The listing builds one solid part. Answer for the finished solid, in the listing's coordinates (mm). Face numbers are marked on the shaded views. A direction names the side the tool comes from. Round coordinates to 2 decimals unless told otherwise and drop trailing zeros. Order: outer loops, then holes, each group sorted by start corner. A loop starts at its lowest first (then second) coordinate and runs counter-clockwise, first axis right, second up. Notation, with made-up numbers: (-21, 37) -> (-15, 37) arc R15 cw to (-15, 50) -> close; hole circle Ø9 at (11, -11). An arc over 180 degrees is marked (long way). Return JSON: item names as keys, results as strings. Group by question number.
(1) The part is cut by section B-B (y = -31). Determine the outline of the cut face in (x, z), plus the area to 3 significant figures.
(2) The part is cut by section D-D (z = 30.5). Determine the outline of the cut face in (x, y).
(3) Consider line 1 (Y direction, x = -22, z = 69.5); line 2 (X direction, y = -21, z = 44.5); line 3 (X direction, y = -56, z = 28.5). Determine where each line is inside the solid, lowest interval first. Write a range as [from, to].
(4) Which of the six approach directions +Z, -Z, +X, -X, +Y, -Y give full straight-line access (tool end or side, diameter ignored) to the marked faces 1 and 2?
(5) The part is cut by section C-C (x = -68). Determine the outline of the cut face in (y, z).
(6) The part is cut by section A-A (z = 38.5). Determine the outline of the cut face in (x, y).
(7) Each of these flat-tipped pins is pushed along its axis until it touches: pin 1 (16 mm diameter, centred on y = -53.5, z = 12.5, fed in from +X); pin 2 (10 mm diameter, centred on x = -61, y = -29.5, fed in from +Z); pin 3 (1 mm diameter, centred on y = -39, z = 10, fed in from +X). Where does it stop, or does it pass through?
(8) Determine the mould class of the marked faces 3, 4, 5 and 6 for opening direction Z: +Z half, -Z half, draft (parallel to the pull), parting line (faces both ways), or undercut.
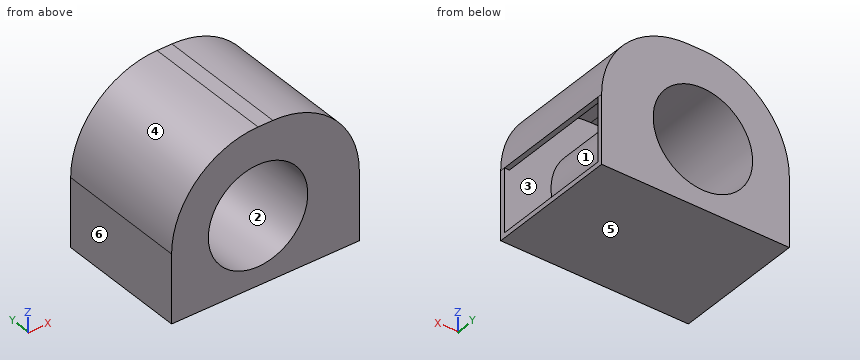
from build123d import *

# Parameters (mm, degrees)
F0_W     = 95.8885699511
F0_H     = 67.4029458314
F1_DEPTH = 78.994
F2_R     = 44.1511376287
F4_D     = 50.8
F5_T     = -2.54


# Not quite as in the source:
# - a shell that OpenCascade refuses in one call is made with other operations: the cavity is built on its own and cut out


with BuildPart() as f1:
    # F0 (on Top) → F1 (new body)
    with BuildSketch(Plane.XY):
        with Locations((-40.1296839118, -48.2643311843)):
            Rectangle(F0_W, F0_H)
    extrude(amount=F1_DEPTH)

    # F2
    f2_edges = [f1.edges().sort_by_distance(p)[0] for p in [
        (-88.073969, -48.264331, 78.994),
        (7.814601, -48.264331, 78.994),
    ]]
    fillet(f2_edges, radius=F2_R)

    # F4 (through all)
    with Locations(Plane.XZ.offset(81.9658041)):
        with Locations((-43.9228312586, 34.8428623713)):
            Hole(F4_D / 2)

    # F5: a shell. OpenCascade refuses it in one call, so the cavity is built on its own and cut out:
    # the body offset inwards by the wall thickness, plus a prism from it out through each open face.
    f5_core = offset(f1.part, amount=F5_T, mode=Mode.PRIVATE)
    f5_exits = [f5_core.faces().sort_by_distance(p)[0] for p in [
        (5.274601, -48.264331, 18.691431),
    ]]
    add(f5_core, mode=Mode.SUBTRACT)
    extrude(f5_exits, amount=-F5_T, mode=Mode.SUBTRACT)


solid = f1.part
Answer below:
{
 "1": {"outline": "(-88.07, 0) -> (7.81, 0) -> (7.81, 2.54) -> (-85.53, 2.54) -> (-85.53, 34.84) arc R41.61 cw to (-43.92, 76.45) -> (-36.34, 76.45) arc R41.61 cw to (5.27, 34.84) -> (7.81, 34.84) arc R44.15 ccw to (-36.34, 78.99) -> (-43.92, 78.99) arc R44.15 ccw to (-88.07, 34.84) -> close; circle Ø55.88 at (-43.92, 34.84); hole circle Ø50.8 at (-43.92, 34.84)", "area": "1,110 mm²"},
 "2": {"outline": "(-88.07, -81.97) -> (-68.95, -81.97) -> (-68.95, -14.56) -> (-88.07, -14.56) -> close; (-18.9, -81.97) -> (7.81, -81.97) -> (7.81, -79.43) -> (-16.32, -79.43) -> (-16.32, -17.1) -> (7.81, -17.1) -> (7.81, -14.56) -> (-18.9, -14.56) -> close; hole (-85.53, -79.43) -> (-71.52, -79.43) -> (-71.52, -17.1) -> (-85.53, -17.1) -> close"},
 "3": {"line 1": "y = [-81.97, -79.43], [-17.1, -14.56]", "line 2": "x = [-87, -84.4], [-70.14, -67.42], [-20.43, -17.7], [4.14, 6.75]", "line 3": "x = [-88.07, -85.53], [-71.13, -68.52], [-19.33, -16.71]"},
 "4": {"face 1": "none", "face 2": "+Y, -Y"},
 "5": {"outline": "(-81.97, 0) -> (-14.56, 0) -> (-14.56, 26.75) -> (-81.97, 26.75) -> close; (-81.97, 42.93) -> (-14.56, 42.93) -> (-14.56, 71.85) -> (-81.97, 71.85) -> close; hole (-79.43, 2.54) -> (-17.1, 2.54) -> (-17.1, 20.67) -> (-79.43, 20.67) -> close; hole (-79.43, 49.02) -> (-17.1, 49.02) -> (-17.1, 68.78) -> (-79.43, 68.78) -> close"},
 "6": {"outline": "(-87.92, -81.97) -> (-69.06, -81.97) -> (-69.06, -14.56) -> (-87.92, -14.56) -> close; (-18.79, -81.97) -> (7.66, -81.97) -> (7.66, -14.56) -> (-18.79, -14.56) -> close; hole (-85.37, -79.43) -> (-71.62, -79.43) -> (-71.62, -17.1) -> (-85.37, -17.1) -> close; hole (-16.22, -79.43) -> (5.11, -79.43) -> (5.11, -17.1) -> (-16.22, -17.1) -> close"},
 "7": {"pin 1": "stops at x = -19.95", "pin 2": "stops at z = 77.31", "pin 3": "stops at x = -30.21"},
 "8": {"face 3": "undercut", "face 4": "+Z half", "face 5": "-Z half", "face 6": "draft"}
}
